Geometry: final body of the model. Coordinates: model frame, mm. Face numbers are marked on the shaded views. A direction names the side the tool comes from. Round coordinates to 2 decimals unless told otherwise and drop trailing zeros. Loops run counter-clockwise (first coordinate to the right, second up) from the corner with the lowest first, then second, coordinate; pieces in that order, holes last. Notation, with made-up numbers: (56, 31) - (63, 31) arc R20 cw to (63, 64) - close; hole circle Ø3 at (57.5, 4). An arc over 180 degrees is marked (long way). Write item = value, one per line. Start each with the question number.
Item 1: Access query for the marked faces 1 and 2. Directions: +Z, -Z, +X, -X, +Y, -Y. A direction counts if a zero-diameter tool reaches every point of the face in a straight line with its end or side. Return the directions, or none.
Item 2: Line query: line 1 (X direction, y = -36.5, z = -157); line 2 (Z direction, x = 15, y = -3); line 3 (Z direction, x = 6.5, y = -11.5). Output: solid intervals per line, ascending. Write a range as from..to.
Item 3: Draft query along Y for the marked faces 3, 4 and 5. Return one class per face: pulls with the +Y half, pulls with the -Y half, needs draft (parallel to the pull), parting line crosses it, or undercut.
Item 4: Section D-D (y = -21.5). Return loops of the section in (x, z).
Item 5: First-contact query: pin 1 (9 mm diameter, centred on x = 14.5, y = -22, fed in from +Z); pin 2 (2 mm diameter, centred on x = 6.5, z = -79.5, fed in from +Y); pin 3 (15 mm diameter, centred on x = 23, y = -16, fed in from -Z); pin 4 (3 mm diameter, centred on y = -27, z = -58, fed in from -X). Flat tips, straight axial feed; report the tip coordinate or a pass-through.
Item 6: Section A-A (z = -15). Return loops of the section in (x, y).
Item 7: Section C-C (z = -157). Return loops of the section in (x, y), plus the area to 3 significant figures.
Item 8: Section B-B (x = 26.5). Return loops of the section in (y, z), plus the area to 3 significant figures.
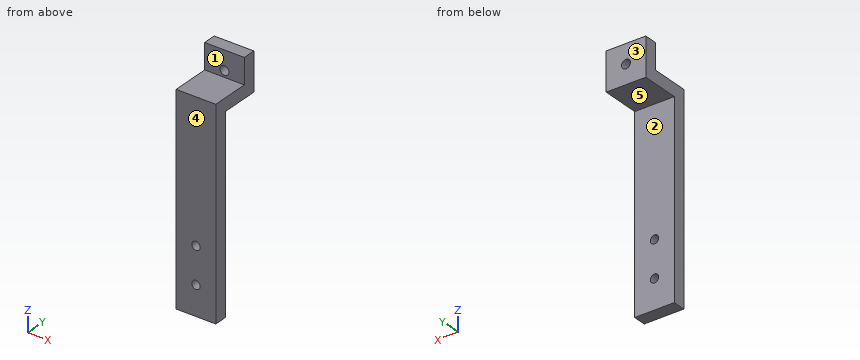
from build123d import *

# Parameters (mm, degrees)
EXTRUDE_THIN1_DEPTH            = 31
SKETCH6_R                      = 3.5
CUT_EXTRUDE1_DEPTH             = 10
SKETCH7_R                      = 3.302
CUT_EXTRUDE3_DEPTH             = 10.16
F_97_0_26_DIAMETER_HOLE1_D     = 6.604
F_97_0_26_DIAMETER_HOLE1_DEPTH = 25.4
F_97_0_26_DIAMETER_HOLE1_TIP   = 1.984041764


with BuildPart() as part:
    # Sketch1 → Extrude-Thin1 (new body)
    with BuildSketch(Plane(origin=(0, 0, 0), x_dir=(0, 0, -1), z_dir=(1, 0, 0))):
        Polygon((0, 0), (30, 0), (30, -29.972), (180, -29.972), (180, -39.972), (20, -39.972), (20, -10), (0, -10), align=None)
    extrude(amount=EXTRUDE_THIN1_DEPTH)

    # Sketch6 → Cut-Extrude1 (cut)
    with BuildSketch(Plane(origin=(0, 0, 0), x_dir=(1, 0, 0), z_dir=(0, 1, 0))):
        with Locations(Location((15.5, 15, 0), (0, 0, 270))):
            Circle(SKETCH6_R)
    extrude(amount=-CUT_EXTRUDE1_DEPTH, mode=Mode.SUBTRACT)

    # Sketch7 → Cut-Extrude3 (cut)
    with BuildSketch(Plane(origin=(0, -29.972, 0), x_dir=(1, 0, 0), z_dir=(0, 1, 0))):
        with Locations(Location((15.494, 157, 0), (0, 0, 270))):
            Circle(SKETCH7_R)
    extrude(amount=-CUT_EXTRUDE3_DEPTH, mode=Mode.SUBTRACT)

    # #97 (0.26) Diameter Hole1
    with Locations(Plane(origin=(0, -29.972, 0), x_dir=(1, 0, 0), z_dir=(0, 1, 0))):
        with Locations((15.494, 128.552)):
            Hole(F_97_0_26_DIAMETER_HOLE1_D / 2, depth=F_97_0_26_DIAMETER_HOLE1_DEPTH)
            with Locations((0, 0, -(F_97_0_26_DIAMETER_HOLE1_DEPTH + F_97_0_26_DIAMETER_HOLE1_TIP / 2))):  # 118° drill point
                Cone(0, F_97_0_26_DIAMETER_HOLE1_D / 2, F_97_0_26_DIAMETER_HOLE1_TIP, mode=Mode.SUBTRACT)


solid = part.part
Taken from the geometry:
q1.face_1 = +Z, +X, -X, -Y
q1.face_2 = -Z, +X, -X, +Y
q2.line_1 = 0..12.19, 18.8..31
q2.line_2 = -30..-18.46, -11.54..0
q2.line_3 = -30..-20
q3.face_3 = pulls with the +Y half
q3.face_4 = pulls with the -Y half
q3.face_5 = needs draft
q4.outline = (0, -30) - (31, -30) - (31, -20) - (0, -20) - close
q5.pin_1 = -20
q5.pin_2 = -29.97
q5.pin_3 = -30
q5.pin_4 = through
q6.outline = (0, -10) - (12, -10) - (12, 0) - (0, 0) - close; (19, -10) - (31, -10) - (31, 0) - (19, 0) - close
q7.outline = (0, -39.97) - (12.19, -39.97) - (12.19, -29.97) - (0, -29.97) - close; (18.8, -39.97) - (31, -39.97) - (31, -29.97) - (18.8, -29.97) - close
q7.area = 244 mm^2
q8.outline = (-39.97, -180) - (-29.97, -180) - (-29.97, -30) - (0, -30) - (0, 0) - (-10, 0) - (-10, -20) - (-39.97, -20) - close
q8.area = 2,100 mm^2
